Here's how the part is built. I have some questions about the finished solid (model axes, mm). A direction names the side the tool comes from. Coordinates: 2 decimals unless noted, no trailing zeros. Write each loop counter-clockwise with the first axis right and the second up, starting at its lowest first coordinate (ties: lowest second). Pieces come first, ordered by that corner, then holes.
```python
from build123d import *

# Parameters (mm, degrees)
SKETCH1_R           = 1.5
SKETCH1_R_2         = 5
SKETCH1_R_3         = 2
BOSS_EXTRUDE1_DEPTH = 5


with BuildPart() as part:
    # Sketch1 → Boss-Extrude1 (new body)
    with BuildSketch(Plane(origin=(0, 0, 0), x_dir=(1, 0, 0), z_dir=(0, 1, 0))):
        with BuildLine():
            Line((-1.571428571, 10.887176505), (67, 20.784609691))
            ThreePointArc((67, 20.784609691), (88.351830916, -10.208344725), (50.75875, -8.412746189))
            ThreePointArc((50.75875, -8.412746189), (46.333095385, -3.17793327), (39.76375, -1.220029725))
            Line((39.76375, -1.220029725), (14.741479919, -1.220029725))
            ThreePointArc((14.741479919, -1.220029725), (11.977316072, -2.05356861), (10.134767445, -4.276270436))
            ThreePointArc((10.134767445, -4.276270436), (-8.707193804, -6.721962218), (-1.571428571, 10.887176505))
        make_face()
        Circle(SKETCH1_R, mode=Mode.SUBTRACT)
        with Locations((70, 0)):
            Circle(SKETCH1_R_2, mode=Mode.SUBTRACT)
        with Locations((70, 12)):
            Circle(SKETCH1_R_3, mode=Mode.SUBTRACT)
        with Locations((82, 0)):
            Circle(SKETCH1_R_3, mode=Mode.SUBTRACT)
        with Locations((70, -12)):
            Circle(SKETCH1_R_3, mode=Mode.SUBTRACT)
        with Locations((58, 0)):
            Circle(SKETCH1_R_3, mode=Mode.SUBTRACT)
    extrude(amount=BOSS_EXTRUDE1_DEPTH)


solid = part.part
```
1) I need wall thicknesses on probe 1 along Z at (x, y) = (70, 3.1); probe 2 along X at (y, z) = (1.6, 0); probe 3 along Z at (x, y) = (69, 0.2). Which ranges of each line are inside material? Lowest first, please.
Values follow:
probe 1: z = -21 to -14, -10 to -5, 5 to 10, 14 to 21
probe 2: x = -11 to -1.5, 1.5 to 56, 60 to 65, 75 to 80, 84 to 91
probe 3: z = -20.98 to -13.73, -10.27 to -4.9, 4.9 to 10.27, 13.73 to 20.98
2) Imagine slicing it at A-A on z = 0. Please give me the cut outline in (x, y), then the cut area to 3 significant figures.
Values follow:
outline: (-11, 0) - (-1.5, 0) - (-1.5, 5) - (-11, 5) - close; (1.5, 0) - (56, 0) - (56, 5) - (1.5, 5) - close; (60, 0) - (65, 0) - (65, 5) - (60, 5) - close; (75, 0) - (80, 0) - (80, 5) - (75, 5) - close; (84, 0) - (91, 0) - (91, 5) - (84, 5) - close
area: 405 mm2
3) Will these pins go through, and if not, where does the flat tip stop? pin 1 (6.5 mm diameter, centred on x = 58, z = 0, fed in from +Y); pin 2 (1.5 mm diameter, centred on x = 54, y = 4.5, fed in from +Z); pin 3 (3 mm diameter, centred on x = 26.5, y = 2, fed in from -Z); pin 4 (3 mm diameter, centred on y = 3.5, z = -9.5, fed in from +X).
Values follow:
pin 1: stops at y = 5
pin 2: stops at z = 14.44
pin 3: stops at z = -15.16
pin 4: stops at x = 89.42
4) On a 3-axis mill with a long thin cutter (end or side, diameter ignored), from which of +Z, -Z, +X, -X, +Y, -Y can I reach the whole of each face in a straight line? I mean faces 4 (the face through (46.41, 2.46, 3.23)), 5 (the face through (83.908, 2.465, -0.601)). Say none if no direction works.
Values follow:
face 4: +Z, +Y, -Y
face 5: +Y, -Y
5) Imagine slicing it at B-B on y = 3.2. Please give me the cut outline in (x, z), then the cut area to 3 significant figures.
Values follow:
outline: (-1.57, -10.89) - (67, -20.78) arc R21 ccw (long way) to (50.76, 8.41) arc R12 cw to (39.76, 1.22) - (14.74, 1.22) arc R5 cw to (10.13, 4.28) arc R11 ccw (long way) to start; hole circle Ø3 at (0, 0); hole circle Ø4 at (58, 0); hole circle Ø10 at (70, 0); hole circle Ø4 at (70, -12); hole circle Ø4 at (70, 12); hole circle Ø4 at (82, 0)
area: 2,380 mm2
6) Imagine slicing it at D-D on z = -12. Please give me the cut outline in (x, y).
Values follow:
outline: (6.14, 0) - (68, 0) - (68, 5) - (6.14, 5) - close; (72, 0) - (87.23, 0) - (87.23, 5) - (72, 5) - close
7) Imagine slicing it at C-C on x = 0. Please give me the cut outline in (y, z), then the cut area to 3 significant figures.
Values follow:
outline: (0, -11.11) - (5, -11.11) - (5, -1.5) - (0, -1.5) - close; (0, 1.5) - (5, 1.5) - (5, 11) - (0, 11) - close
area: 95.6 mm2
8) We'd pull the mould along X, two halves only. Please class faces 1 (the face through (32.234, 2.465, -15.767)), 2 (the face through (12.01, 2.46, 2.03)), 3 (the face through (52, 0, 0)): pulls with the +X half, pulls with the -X half, needs draft (parallel to the pull), parting line crosses it, or undercut.
Values follow:
face 1: pulls with the -X half
face 2: undercut
face 3: needs draft
